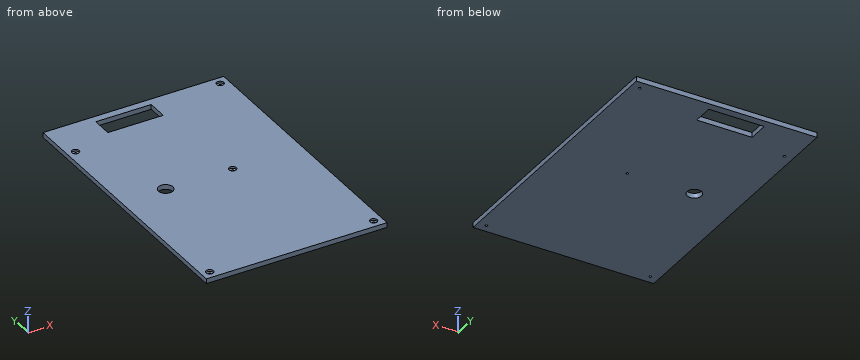
from build123d import *

# Parameters (mm, degrees)
SKETCH1_W                      = 150
SKETCH1_H                      = 230
BOSS_EXTRUDE1_DEPTH            = 4
TAP_DRILL_FOR_M2_5X0_45_TAP2_D = 2.05
SKETCH8_R                      = 3.025
CUT_EXTRUDE2_DEPTH             = 1.5
CUT_EXTRUDE3_REACH             = 139.354
SKETCH9_W                      = 46
SKETCH9_H                      = 17
CUT_EXTRUDE3_DIRECTION_2_DEPTH = 138.353558381
CUT_EXTRUDE4_REACH             = 139.354
SKETCH10_R                     = 6


with BuildPart() as part:
    # Sketch1 → Boss-Extrude1 (new body)
    with BuildSketch(Plane.XY):
        Rectangle(SKETCH1_W, SKETCH1_H)
    extrude(amount=BOSS_EXTRUDE1_DEPTH)

    # Tap Drill for M2.5x0.45 Tap2 (through all)
    with Locations(Plane(origin=(68, 108, 0), x_dir=(-1, 0, 0), z_dir=(0, 0, -1))):
        with Locations((0, 0), (136, -27), (0, -216), (136, -216), (51, -104)):
            Hole(TAP_DRILL_FOR_M2_5X0_45_TAP2_D / 2)

    # Sketch8 → Cut-Extrude2 (cut)
    with BuildSketch(Plane.XY.offset(4)):
        with Locations((-68, 81)):
            Circle(SKETCH8_R)
        with Locations((68, 108)):
            Circle(SKETCH8_R)
        with Locations((-68, -108)):
            Circle(SKETCH8_R)
        with Locations((68, -108)):
            Circle(SKETCH8_R)
        with Locations((17, 4)):
            Circle(SKETCH8_R)
    extrude(amount=-CUT_EXTRUDE2_DEPTH, mode=Mode.SUBTRACT)

    # Sketch9 → Cut-Extrude3 (cut, up to next)
    with BuildSketch(Plane.XY.offset(4), mode=Mode.PRIVATE) as cut_extrude3_sk1:
        with Locations((-12, 100)):
            Rectangle(SKETCH9_W, SKETCH9_H)
    cut_extrude3_tool1 = extrude(cut_extrude3_sk1.sketch, amount=-CUT_EXTRUDE3_REACH, mode=Mode.PRIVATE) & part.part
    add(cut_extrude3_tool1.solids().sort_by_distance((-12, 100, 4))[0], mode=Mode.SUBTRACT)

    # Sketch9 → Cut-Extrude3 direction 2 (cut)
    with BuildSketch(Plane.XY.offset(4)):
        with Locations((-12, 100)):
            Rectangle(SKETCH9_W, SKETCH9_H)
    extrude(amount=CUT_EXTRUDE3_DIRECTION_2_DEPTH, mode=Mode.SUBTRACT)

    # Sketch10 → Cut-Extrude4 (cut, up to next)
    with BuildSketch(Plane.XY.offset(4), mode=Mode.PRIVATE) as cut_extrude4_sk1:
        with Locations((-38.202297392, 4.692384057)):
            Circle(SKETCH10_R)
    cut_extrude4_tool1 = extrude(cut_extrude4_sk1.sketch, amount=-CUT_EXTRUDE4_REACH, mode=Mode.PRIVATE) & part.part
    add(cut_extrude4_tool1.solids().sort_by_distance((-38.202297, 4.692384, 4))[0], mode=Mode.SUBTRACT)


solid = part.part
Could you check a few things on this model? Use its own coordinates, in mm. Give positions to 0.01 mm unless a question says otherwise; leave off trailing zeros. Write each loop counter-clockwise with the first axis right and the second up, starting at its lowest first coordinate (ties: lowest second). Pieces come first, ordered by that corner, then holes. Notation, with made-up numbers: (11, 87) -> (30, 87) arc R21 ccw to (30, 95) -> close; hole circle Ø1 at (-5.5, 45.25). An arc over 180 degrees is marked (long way). Write each question's results on one line, items separated by ' | '. Start each with the question number.
Q1. Suppose I cut it at A-A, the plane x = -18. List the corners of the cut face in (y, z) for me.
Q2. Suppose I cut it at B-B, the plane z = 1.5. List the corners of the cut face in (x, y) for me (3 decimals), and give its area (3 significant figures).
Q3. I need wall thicknesses on probe 1 along Y at (x, z) = (-68, 1.85) (3 decimals); probe 2 along X at (y, z) = (108, 1.5) (3 decimals); probe 3 along Y at (x, z) = (68, 3.5) (3 decimals). Which ranges of each line are inside material? Lowest first, please.
Q4. I'm going to push a flat-ended pin straight in: pin 1 Ø5.5 at (x, y) = (17, 4) entering from +Z. Where does the tip first touch, or does it pass through?
Outcome:
1) outline: (-115, 0) -> (91.5, 0) -> (91.5, 4) -> (-115, 4) -> close; (108.5, 0) -> (115, 0) -> (115, 4) -> (108.5, 4) -> close
2) outline: (-75, -115) -> (75, -115) -> (75, 115) -> (-75, 115) -> close; hole circle Ø2.05 at (-68, -108); hole circle Ø2.05 at (-68, 81); hole circle Ø12 at (-38.202, 4.692); hole (-35, 91.5) -> (11, 91.5) -> (11, 108.5) -> (-35, 108.5) -> close; hole circle Ø2.05 at (17, 4); hole circle Ø2.05 at (68, -108); hole circle Ø2.05 at (68, 108) | area: 33,600 mm2
3) probe 1: -115 to -109.025, -106.975 to 79.975, 82.025 to 115 | probe 2: -75 to -35, 11 to 66.975, 69.025 to 75 | probe 3: -115 to -111.025, -104.975 to 104.975, 111.025 to 115
4) pin 1: z = 2.5
